Part model, mm, in its own coordinate system. A direction names the side the tool comes from. Coordinates: 2 decimals unless noted, no trailing zeros. Loops run counter-clockwise (first coordinate to the right, second up) from the corner with the lowest first, then second, coordinate; pieces in that order, holes last. Notation, with made-up numbers: (48, -27.5) - (53, -27.5) arc R19 cw to (53, -15.5) - close; hole circle Ø4 at (66, 86.5). An arc over 180 degrees is marked (long way). Use a Markdown table: item, result. Add a question column.
1) Drop flat-ended pins along their axis: P1, Ø1.5, axis at y = 31.5, z = 12.5, coming from the +X side; P2, Ø4, axis at y = 36, z = 9.5, coming from the +X side. Give the stop position or say it passes through.
2) Band-saw the part on A-A (y = 35). Give the cut face in (x, z).
3) Band-saw the part on C-C (x = 111.75). Give the cut face in (y, z), plus the area to 3 significant figures.
4) Tool access for faces 1 (the face through (105.873, 29.091, 4.258)), 2 (the face through (110, 33, 0)), 3 (the face through (107, 30, 27.601)): list every direction of +Z, -Z, +X, -X, +Y, -Y with a clear straight run to the whole face (end or side of a thin tool).
5) Band-saw the part on B-B (z = 25). Give the cut face in (x, y), plus the area to 3 significant figures.
6) Probe probe 1 along Z at (x, y) = (108, 28.25); probe 2 along Y at (x, z) = (107.5, 13); probe 3 along X at (y, z) = (28.5, 18). List the from-to ranges inside material, lowest first. Write a range as [from, to].
7) Band-saw the part on D-D (y = 27.5). Give the cut face in (x, z), plus the area to 3 significant figures.
from build123d import *

# Parameters (mm, degrees)
SKETCH1_R           = 5.926666667
BOSS_EXTRUDE1_DEPTH = 8.636
SKETCH2_R           = 6.326666667
BOSS_EXTRUDE2_DEPTH = 18.965333333
BOSS_EXTRUDE3_DEPTH = 3.386666667


with BuildPart() as part:
    # Sketch1 → Boss-Extrude1 (new body)
    with BuildSketch(Plane.XY):
        with Locations((110.576144023, 32.69693519)):
            Circle(SKETCH1_R)
    extrude(amount=BOSS_EXTRUDE1_DEPTH)

    # Sketch2 → Boss-Extrude2 (add)
    with BuildSketch(Plane.XY.offset(8.636)):
        with Locations((110.576144023, 32.69693519)):
            Circle(SKETCH2_R)
    extrude(amount=BOSS_EXTRUDE2_DEPTH)

    # Sketch3 → Boss-Extrude3 (add)
    with BuildSketch(Plane.XY.offset(27.601333333)):
        with BuildLine():
            Line((104.842236757, 35.37070006), (107.984893057, 30.88252173))
            Line((107.984893057, 30.88252173), (111.127549356, 26.3943434))
            ThreePointArc((111.127549356, 26.3943434), (115.240651974, 28.422701143), (116.90281069, 32.69693519))
            ThreePointArc((116.90281069, 32.69693519), (111.945485314, 38.873634595), (104.842236757, 35.37070006))
        make_face()
    extrude(amount=BOSS_EXTRUDE3_DEPTH)


solid = part.part
Answer block:
| question | item | result |
|---|---|---|
| 1 | P1 | x = 116.89 |
| 1 | P2 | x = 116.77 |
| 2 | outline | (104.68, 8.64) - (105.12, 8.64) - (105.12, 0) - (116.04, 0) - (116.04, 8.64) - (116.47, 8.64) - (116.47, 30.99) - (105.1, 30.99) - (105.1, 27.6) - (104.68, 27.6) - close |
| 3 | outline | (26.48, 8.64) - (26.89, 8.64) - (26.89, 0) - (38.51, 0) - (38.51, 8.64) - (38.91, 8.64) - (38.91, 30.99) - (26.48, 30.99) - close |
| 3 | area | 378 mm2 |
| 4 | face 1 | -Z |
| 4 | face 2 | -Z, +X, -X, +Y, -Y |
| 4 | face 3 | +Z, -X, -Y |
| 5 | outline | circle Ø12.65 at (110.58, 32.7) |
| 5 | area | 126 mm2 |
| 6 | probe 1 | [0, 27.6] |
| 6 | probe 2 | [27.17, 38.23] |
| 6 | probe 3 | [105.84, 115.31] |
| 7 | outline | (106.97, 8.64) - (107.73, 8.64) - (107.73, 0) - (113.43, 0) - (113.43, 8.64) - (114.18, 8.64) - (114.18, 30.99) - (110.35, 30.99) - (110.35, 27.6) - (106.97, 27.6) - close |
| 7 | area | 199 mm2 |
